The listing builds one solid part. Answer for the finished solid, in the listing's coordinates (mm). A direction names the side the tool comes from. Coordinates: 2 decimals unless noted, no trailing zeros. Loops run counter-clockwise (first coordinate to the right, second up) from the corner with the lowest first, then second, coordinate; pieces in that order, holes last. Notation, with made-up numbers: (12, 12) -> (68, 12) arc R26 cw to (68, 36) -> close; hole circle Ø8 at (71.5, 44.5). An arc over 180 degrees is marked (long way). Answer in a Markdown table with one row per item.
Autodesk Inventor part; units mm, degrees
ref_plane "YZ Plane" through (0, 0, 0) normal (1, 0, 0) x (0, 1, 0)
ref_plane "XZ Plane" through (0, 0, 0) normal (0, 1, 0) x (-1, 0, 0)
ref_plane "XY Plane" through (0, 0, 0) normal (0, 0, 1) x (1, 0, 0)
sketch "Szkic1" plane through (0, 0, 0) normal (1, 0, 0) x (0, 1, 0)
  line L0 (10, 15) -> (-30, 15)
  line L1 (-30, 15) -> (-30, -35)
  line L2 (-30, -35) -> (10, 15)
  point P0 (0, 0)
  dimension "d0" = 40
  dimension "d1" = 50
extrude "Wyciągnięcie proste1" add sketch "Szkic1" along normal blind 150
shell "Skorupa2" thickness 5 removed faces 1 at (50, -3.3333, 15)
properties part number "sumo_module_shield"
Item 1: A cutting plane is placed at C-C, the plane x = 44.5. Determine the outline of the cut face in (y, z).
Findings below:
| item | result |
|---|---|
| outline | (-30, -35) -> (10, 15) -> (3.6, 15) -> (-25, -20.75) -> (-25, 15) -> (-30, 15) -> close |
Item 2: Flat-ended cylindrical pins translate along their axes: pin 1 Ø18 at (x, z) = (40.5, -9.5) entering from +Y; pin 2 Ø6 at (x, y) = (126, -5.5) entering from +Z; pin 3 Ø10 at (x, z) = (121, 1) entering from +Y; pin 4 Ø6 at (y, z) = (-11, -7) entering from -X. Find the tip coordinate at first contact, or state that the pin passes through.
Findings below:
| item | result |
|---|---|
| pin 1 | stops at y = -2.4 |
| pin 2 | stops at z = 7.38 |
| pin 3 | stops at y = 2.8 |
| pin 4 | stops at x = 0 |
Item 3: Find the intervals of material crossed by probe 1 along X at (y, z) = (-18.5, 10); probe 2 along Z at (x, y) = (136, -26); probe 3 along Y at (x, z) = (45, 7), in increasing order.
Findings below:
| item | result |
|---|---|
| probe 1 | x = 0 to 5, 145 to 150 |
| probe 2 | z = -30 to 15 |
| probe 3 | y = -30 to -25, -2.8 to 3.6 |
Item 4: Determine the mould class of faces 1 (the face through (5, -14, 1)), 2 (the face through (150, -15, -4)), 3 (the face through (74, -30, -10)), 4 (the face through (145, -14, 1)) for opening direction X: +X half, -X half, draft (parallel to the pull), parting line (faces both ways), or undercut.
Findings below:
| item | result |
|---|---|
| face 1 | undercut |
| face 2 | +X half |
| face 3 | draft |
| face 4 | undercut |
Item 5: A cutting plane is placed at B-B, the plane y = -9. Determine the outline of the cut face in (x, z).
Findings below:
| item | result |
|---|---|
| outline | (0, -8.75) -> (150, -8.75) -> (150, 15) -> (145, 15) -> (145, -0.75) -> (5, -0.75) -> (5, 15) -> (0, 15) -> close |
Item 6: A cutting plane is placed at D-D, the plane z = -25. Determine the outline of the cut face in (x, y).
Findings below:
| item | result |
|---|---|
| outline | (0, -30) -> (150, -30) -> (150, -22) -> (0, -22) -> close |
Item 7: A tool of negligible diameter and unlimited length cuts with its end or side. For faces 5 (the face through (74.02, -10.9, -3.12)), 6 (the face through (74, -10, -10)), from which of +Z, -Z, +X, -X, +Y, -Y can it reach the whole face along a straight path? Write none if from no direction.
Findings below:
| item | result |
|---|---|
| face 5 | +Z |
| face 6 | -Z, +X, -X, +Y |
Item 8: A cutting plane is placed at A-A, the plane z = -14. Determine the outline of the cut face in (x, y), plus the area to 3 significant figures.
Findings below:
| item | result |
|---|---|
| outline | (0, -30) -> (150, -30) -> (150, -13.2) -> (0, -13.2) -> close; hole (5, -25) -> (145, -25) -> (145, -19.6) -> (5, -19.6) -> close |
| area | 1,760 mm2 |
